```python
from build123d import *

# Parameters (mm, degrees)
SKETCH1_W           = 44
SKETCH1_H           = 44
BOSS_EXTRUDE1_DEPTH = 106.47
SKETCH5_R           = 15
CUT_EXTRUDE2_DEPTH  = 106.47
SKETCH10_R          = 2.5
CUT_EXTRUDE9_DEPTH  = 1.9


with BuildPart() as part:
    # Sketch1 → Boss-Extrude1 (new body)
    with BuildSketch(Plane.XY):
        Rectangle(SKETCH1_W, SKETCH1_H)
    extrude(amount=BOSS_EXTRUDE1_DEPTH)

    # Sketch5 → Cut-Extrude2 (cut)
    with BuildSketch(Plane(origin=(0, 0, 0), x_dir=(-1, 0, 0), z_dir=(0, 0, -1))):
        Circle(SKETCH5_R)
    extrude(amount=-CUT_EXTRUDE2_DEPTH, mode=Mode.SUBTRACT)

    # Sketch10 → Cut-Extrude9 (cut)
    with BuildSketch(Plane.ZY.offset(22)):
        with Locations((30.2, 3.5)):
            Circle(SKETCH10_R)
        with Locations((76.2, 3.5)):
            Circle(SKETCH10_R)
        with Locations((53.2, -21.499217988)):
            Circle(SKETCH10_R)
    cut_extrude9 = extrude(amount=-CUT_EXTRUDE9_DEPTH, mode=Mode.SUBTRACT)

    # Mirror1: Cut-Extrude9 across plane
    add(cut_extrude9.mirror(Plane(origin=(0, 0, 0), x_dir=(0, 0, 1), z_dir=(1, 0, 0))), mode=Mode.SUBTRACT)


solid = part.part
```
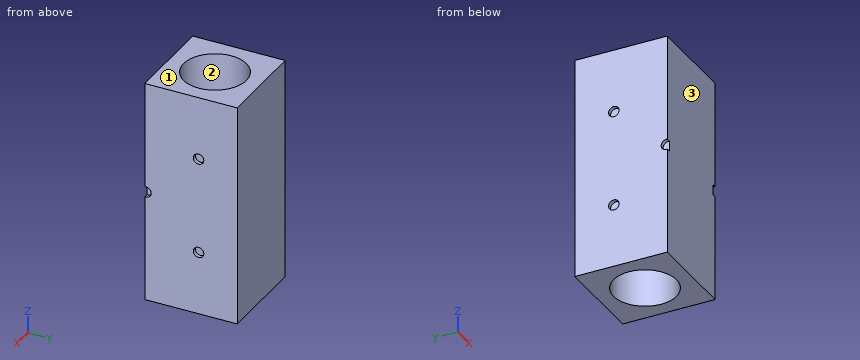
Geometry check sheet. Reference: the model listing, model coordinates, mm. Face numbers are marked on the shaded views. Give positions to 0.01 mm unless a question says otherwise; leave off trailing zeros. Loops run counter-clockwise (first coordinate to the right, second up) from the corner with the lowest first, then second, coordinate; pieces in that order, holes last. Notation, with made-up numbers: M 79,86 L 128,86 A11 cw 128,92 Z; hole C 27.5,-28 d10. An arc over 180 degrees is marked long. Answer as CSV lines item,"result".
Item 1: Material ranges on line 1 (Y direction, x = 21.6, z = 76.2); line 2 (Y direction, x = -21.35, z = 53.2); line 3 (X direction, y = -3.5, z = 18.5), recorded low to high.
Values:
line 1,"y = -22 to 1, 6 to 22"
line 2,"y = -19 to 22"
line 3,"x = -22 to -14.59, 14.59 to 22"
Item 2: Cross-section at A-A on x = 0. Record the cut outline in (y, z).
Values:
outline,"M -22,0 L -15,0 L -15,106.47 L -22,106.47 Z; M 15,0 L 22,0 L 22,106.47 L 15,106.47 Z"
Item 3: Depth check by flat-ended pin: P1, Ø0.9, axis at y = -20.5, z = 53.5, coming from the +X side; P2, Ø4.5, axis at y = -21.5, z = 53.2, coming from the -X side. Enter the tip coordinate at first touch or a pass-through.
Values:
P1,"stops at x = 20.1"
P2,"stops at x = -20.1"
Item 4: Cross-section at B-B on z = 53.2. Record the cut outline in (x, y).
Values:
outline,"M -22,-19 L -20.1,-19 L -20.1,-22 L 20.1,-22 L 20.1,-19 L 22,-19 L 22,22 L -22,22 Z; hole C 0,0 d30"
Item 5: Release check for a two-part mould opening along Y. For the marked faces 1, 2 and 3 record: pulls with the +Y half, pulls with the -Y half, needs draft (parallel to the pull), parting line crosses it, or undercut.
Values:
face 1,"needs draft"
face 2,"undercut"
face 3,"pulls with the -Y half"
Item 6: Cross-section at D-D on z = 76.2. Record the cut outline in (x, y).
Values:
outline,"M -22,-22 L 22,-22 L 22,1 L 20.1,1 L 20.1,6 L 22,6 L 22,22 L -22,22 L -22,6 L -20.1,6 L -20.1,1 L -22,1 Z; hole C 0,0 d30"
Item 7: Cross-section at C-C on y = 3.5. Record the cut outline in (x, z), and give its area (3 significant figures).
Values:
outline,"M -22,0 L -14.59,0 L -14.59,106.47 L -22,106.47 L -22,78.7 L -20.1,78.7 L -20.1,73.7 L -22,73.7 L -22,32.7 L -20.1,32.7 L -20.1,27.7 L -22,27.7 Z; M 14.59,0 L 22,0 L 22,27.7 L 20.1,27.7 L 20.1,32.7 L 22,32.7 L 22,73.7 L 20.1,73.7 L 20.1,78.7 L 22,78.7 L 22,106.47 L 14.59,106.47 Z"
area,"1,540 mm²"
